Source: CAD feature listing. Evaluate the final solid. Frame: model axes, mm. A direction names the side the tool comes from. Round coordinates to 2 decimals unless told otherwise and drop trailing zeros. Order: outer loops, then holes, each group sorted by start corner. A loop starts at its lowest first (then second) coordinate and runs counter-clockwise, first axis right, second up. Notation, with made-up numbers: (11.5, 73) - (62.5, 73) arc R10 cw to (62.5, 77) - close; hole circle Ø8 at (83.5, -37). An arc over 180 degrees is marked (long way). Return JSON: item names as keys, results as strings. Group by question number.
1) Section D-D, the plane z = -4. Return loops of the section in (x, y).
2) Section B-B, the plane z = -73. Return loops of the section in (x, y), plus the area to 3 significant figures.
3) Section C-C, the plane y = 12.5. Return loops of the section in (x, z).
4) Contact query for flat-ended pins moving along their axis: P1, Ø10.5, axis at x = 11.5, y = 9, coming from the -Z side; P2, Ø6, axis at x = -50.5, y = 10.5, coming from the +Z side; P3, Ø5, axis at x = 56, z = -2, coming from the +Y side. Output: stop coordinate, or through.
5) Access query for faces 1 (the flat face through (-52.32, 8.41, 51.56)), 2 (the flat face through (-46.5, 8, -82)), 3 (the flat face through (-51.5, 7, -83)). Directions: +Z, -Z, +X, -X, +Y, -Y. A direction counts if a zero-diameter tool reaches every point of the face in a straight line with its end or side. Return the directions, or none.
6) Ray query, line 1 (X direction, y = 0.7, z = 10); line 2 (X direction, y = 13, z = -45); line 3 (Y direction, x = -55, z = 29). Return the intervals inside material, ascending. Write a range as from..to.
7) Section A-A, the plane x = -30. Return loops of the section in (y, z).
```python
from build123d import *

# Parameters (mm, degrees)
BOSS_EXTRUDE1_DEPTH = 2
EXTRUDE_THIN3_DEPTH = 15
SKETCH3_W           = 93
SKETCH3_H           = 13
CUT_EXTRUDE1_DEPTH  = 5
SKETCH5_R           = 50
CUT_EXTRUDE2_DEPTH  = 2
BOSS_EXTRUDE2_DEPTH = 2.5
SKETCH4_3_R         = 2.65
CUT_EXTRUDE3_DEPTH  = 2.5


with BuildPart() as part:
    # Sketch1 → Boss-Extrude1 (new body)
    with BuildSketch(Plane(origin=(0, 0, 0), x_dir=(1, 0, 0), z_dir=(0, 1, 0))):
        Polygon((-46.5, 140), (46.5, 140), (46.5, 21.653994317), (65, 0), (65, -37.732612768), (40, -65), (-40, -65), (-65, -37.732612768), (-65, 0), (-46.5, 21.653994317), align=None)
    extrude(amount=BOSS_EXTRUDE1_DEPTH)

    # Sketch1<6> → Extrude-Thin3 (add)
    with BuildSketch(Plane(origin=(0, 0, 0), x_dir=(1, 0, 0), z_dir=(0, 1, 0))):
        Polygon((-51.5, 145), (51.5, 145), (51.5, 23.49902712), (70, 1.845032803), (70, -39.677811978), (42.199217545, -70), (-42.199217545, -70), (-70, -39.677811978), (-70, 1.845032803), (-51.5, 23.49902712), align=None)
        Polygon((-46.5, 140), (46.5, 140), (46.5, 21.653994317), (65, 0), (65, -37.732612768), (40, -65), (-40, -65), (-65, -37.732612768), (-65, 0), (-46.5, 21.653994317), align=None, mode=Mode.SUBTRACT)
    extrude(amount=EXTRUDE_THIN3_DEPTH)

    # Sketch3 → Cut-Extrude1 (cut)
    with BuildSketch(Plane.XY.offset(-140)):
        with Locations((0, 8.5)):
            Rectangle(SKETCH3_W, SKETCH3_H)
    extrude(amount=-CUT_EXTRUDE1_DEPTH, mode=Mode.SUBTRACT)

    # Sketch5 → Cut-Extrude2 (cut)
    with BuildSketch(Plane(origin=(0, 2, 0), x_dir=(1, 0, 0), z_dir=(0, 1, 0))):
        with Locations(Location((0, -10, 0), (0, 0, 270))):
            Circle(SKETCH5_R)
    extrude(amount=-CUT_EXTRUDE2_DEPTH, mode=Mode.SUBTRACT)

    # Sketch4 → Boss-Extrude2 (add)
    with BuildSketch(Plane(origin=(0, 15, 0), x_dir=(1, 0, 0), z_dir=(0, 1, 0))):
        with BuildLine():
            Line((-0.5, -5), (0.5, -5))
            ThreePointArc((0.5, -5), (3.681980515, -6.318019485), (5, -9.5))
            Line((5, -9.5), (5, -70))
            Line((5, -70), (-5, -70))
            Line((-5, -70), (-5, -9.5))
            ThreePointArc((-5, -9.5), (-3.681980515, -6.318019485), (-0.5, -5))
        make_face()
    extrude(amount=BOSS_EXTRUDE2_DEPTH)

    # Sketch4<3> → Cut-Extrude3 (cut)
    with BuildSketch(Plane(origin=(0, 15, 0), x_dir=(1, 0, 0), z_dir=(0, 1, 0))):
        with Locations(Location((0, -10, 0), (0, 0, 270))):
            Circle(SKETCH4_3_R)
    extrude(amount=CUT_EXTRUDE3_DEPTH, mode=Mode.SUBTRACT)


solid = part.part
```
Geometry check:
{
 "1": {"outline": "(-68.16, 0) - (-48, 0) - (-48, 2) - (-61.58, 2) - (-61.58, 15) - (-68.16, 15) - close; (48, 0) - (68.16, 0) - (68.16, 15) - (61.58, 15) - (61.58, 2) - (48, 2) - close"},
 "2": {"outline": "(-51.5, 0) - (51.5, 0) - (51.5, 15) - (46.5, 15) - (46.5, 2) - (-46.5, 2) - (-46.5, 15) - (-51.5, 15) - close", "area": "336 mm2"},
 "3": {"outline": "(-70, -1.85) - (-51.5, -23.5) - (-51.5, -145) - (-46.5, -145) - (-46.5, -21.65) - (-65, 0) - (-65, 37.73) - (-40, 65) - (40, 65) - (65, 37.73) - (65, 0) - (46.5, -21.65) - (46.5, -145) - (51.5, -145) - (51.5, -23.5) - (70, -1.85) - (70, 39.68) - (42.2, 70) - (-42.2, 70) - (-70, 39.68) - close"},
 "4": {"P1": "z = 65", "P2": "z = 64.22", "P3": "y = 2"},
 "5": {"face 1": "+Y", "face 2": "-Z, +Y", "face 3": "-Z, -X, +Y, -Y"},
 "6": {"line 1": "-70..-50, 50..70", "line 2": "-51.5..-46.5, 46.5..51.5", "line 3": "0..2"},
 "7": {"outline": "(0, -145) - (2, -145) - (2, -30) - (0, -30) - close; (0, 50) - (2, 50) - (2, 65) - (15, 65) - (15, 70) - (0, 70) - close"}
}
